CAD build for the part. Positions are in the model's coordinates, mm. A direction names the side the tool comes from. Round coordinates to 2 decimals unless told otherwise and drop trailing zeros. Loops run counter-clockwise (first coordinate to the right, second up) from the corner with the lowest first, then second, coordinate; pieces in that order, holes last.
from build123d import *

# Parameters (mm, degrees)
SKETCH001_R  = 2.5
PAD001_DEPTH = 5
SKETCH_W     = 12
SKETCH_H     = 18
SKETCH_R     = 2
PAD_DEPTH    = 5


with BuildPart() as pad001:
    # Sketch001 → Pad001 (new body, symmetric)
    with BuildSketch(Plane.YZ):
        with BuildLine():
            Line((0, 0), (10, 0))
            Line((10, 0), (10, 16))
            ThreePointArc((10, 16), (5, 21), (0, 16))
            Line((0, 16), (0, 0))
        make_face()
        with Locations((5, 16)):
            Circle(SKETCH001_R, mode=Mode.SUBTRACT)
    extrude(amount=PAD001_DEPTH, both=True)


with BuildPart() as fusion:
    # Sketch → Pad (new body)
    with BuildSketch(Plane.XY):
        with Locations((0, 9)):
            Rectangle(SKETCH_W, SKETCH_H)
        with Locations((0, 14)):
            Circle(SKETCH_R, mode=Mode.SUBTRACT)
    extrude(amount=PAD_DEPTH)

    # Fusion: union Pad001
    add(pad001.part)


solid = fusion.part
Item 1: Cut at C-C (z = 2). List the corners of the cut face in (x, y).
Verdict:
outline: (-6, 0) - (6, 0) - (6, 18) - (-6, 18) - close; hole circle Ø4 at (0, 14)
Item 2: Cut at A-A (x = 0). List the corners of the cut face in (y, z).
Verdict:
outline: (0, 0) - (12, 0) - (12, 5) - (10, 5) - (10, 16) arc R5 ccw to (0, 16) - close; (16, 0) - (18, 0) - (18, 5) - (16, 5) - close; hole circle Ø5 at (5, 16)
Item 3: 3-axis set-ups, long thin cutter, end or side, ignore diameter. For faces 1 (the flat face through (-5, 5, 11)), 2 (the flat face through (-6, 9, 2)), 3 (the flat face through (0, 10, 10)): which of +Z, -Z, +X, -X, +Y, -Y reach the whole face in a straight line?
Verdict:
face 1: +Z, -X, +Y, -Y
face 2: +Z, -Z, -X, +Y, -Y
face 3: +Z, +X, -X, +Y
Item 4: Flat gauge pins, fed straight in: P1, Ø2.5, axis at x = 0, y = 14, coming from the +Z side; P2, Ø5, axis at x = -4, z = 16.5, coming from the +Y side; P3, Ø3, axis at y = 3.5, z = 11.5, coming from the +X side; P4, Ø8, axis at y = 9, z = 16.5, coming from the -X side. Where does each tip first touch, or does it go through?
Verdict:
P1: passes through
P2: stops at y = 10
P3: stops at x = 5
P4: stops at x = -5
Item 5: Wall check: L1, parallel to Y at x = 0, z = 1.2; L2, parallel to Z at x = -1, y = 5; L3, parallel to Z at x = -1, y = 11. Give the ranges that are in metal, low to high.
Verdict:
L1: y = 0 to 12, 16 to 18
L2: z = 0 to 13.5, 18.5 to 21
L3: z = 0 to 5
Item 6: Cut at B-B (y = 5). List the corners of the cut face in (x, z).
Verdict:
outline: (-6, 0) - (6, 0) - (6, 5) - (5, 5) - (5, 13.5) - (-5, 13.5) - (-5, 5) - (-6, 5) - close; (-5, 18.5) - (5, 18.5) - (5, 21) - (-5, 21) - close
Item 7: Mould opens along X. For faces 4 (the cylindrical face through (0, 16, 2)), 5 (the flat face through (0, 11, 5)), 6 (the flat face through (5, 5, 11)) say: released by +X, released by -X, zero draft, split by the parting line, or undercut.
Verdict:
face 4: undercut
face 5: zero draft
face 6: released by +X
Item 8: Cut at D-D (x = -3.5). List the corners of the cut face in (y, z), plus the area to 3 significant figures.
Verdict:
outline: (0, 0) - (18, 0) - (18, 5) - (10, 5) - (10, 16) arc R5 ccw to (0, 16) - close; hole circle Ø5 at (5, 16)
area: 220 mm2
